```python
from build123d import *

# Parameters (mm, degrees)
F3_DEPTH    = 6.5
F4_T1_DEPTH = 87.9231463955
F4_T3_DEPTH = 86.4923799402
F5_R        = 35
F6_T        = -1.25


# Not quite as in the source:
# - a fillet or chamfer that OpenCascade refuses, or shapes differently, is made with other operations: its cross-section is extruded or revolved along the edge and cut away or added


with BuildPart() as f3:
    # F2 (on Front) → F3 (new body)
    with BuildSketch(Plane.XZ):
        Polygon((0, 19.5199243858), (20, 0), (215, 0), (215, 7.5), (23.0533679898, 7.5), (0, 30), align=None)
    extrude(amount=F3_DEPTH)

    # F4: fillet of radius 40 on 2 edges, made by hand

    # F4_s2 → F4_t1 (cut)
    with BuildSketch(Plane.XZ.offset(-40.7115731978)):
        with BuildLine():
            ThreePointArc((8.3460077876, 11.374252339), (21.2020218527, 2.9525310821), (36.2846292791, 0))
            Line((36.2846292791, 0), (20, 0))
            Line((20, 0), (8.3460077876, 11.374252339))
        make_face()
    extrude(amount=F4_T1_DEPTH, mode=Mode.SUBTRACT)

    # F4_s4 → F4_t3 (cut)
    with BuildSketch(Plane.XZ.offset(-39.9961899701)):
        with BuildLine():
            ThreePointArc((11.4492084149, 8.345540259), (4.0262452257, 18.2748088699), (0, 30))
            Line((0, 30), (0, 19.5199243858))
            Line((0, 19.5199243858), (11.4492084149, 8.345540259))
        make_face()
    extrude(amount=F4_T3_DEPTH, mode=Mode.SUBTRACT)

    # F5
    f5_edges = [f3.edges().sort_by_distance(p)[0] for p in [
        (23.053368, -3.25, 7.5),
    ]]
    fillet(f5_edges, radius=F5_R)

    # F6
    f6_openings = [f3.faces().sort_by_distance(p)[0] for p in [
        (6.428062, -3.25, 23.726235),
        (24.105137, -3.25, 10.083465),
        (126.151209, -3.25, 7.5),
        (215, -3.25, 3.75),
    ]]
    offset(amount=F6_T, openings=f6_openings)


solid = f3.part
```
Build history of the part. All positions in model axes, mm. A direction names the side the tool comes from. Round coordinates to 2 decimals unless told otherwise and drop trailing zeros. Write each loop counter-clockwise with the first axis right and the second up, starting at its lowest first coordinate (ties: lowest second). Pieces come first, ordered by that corner, then holes. Notation, with made-up numbers: (89, -17.5) - (147, -17.5) arc R16 ccw to (147, -12.5) - close; hole circle Ø8 at (-26.5, 65.25). An arc over 180 degrees is marked (long way). Write each question's results on one line, items separated by ' | '. Start each with the question number.
Item 1: Saw through at A-A (x = 93). Write the cut outline in (y, z), and give its area (4 significant figures).
Item 2: Wall check: L1, parallel to Z at x = 160, y = -2; L2, parallel to Z at x = 69, y = -0.5; L3, parallel to X at y = -5.5, z = 13. Give the ranges that are in metal, low to high. Write a range as [from, to].
Item 3: Drop flat-ended pins along their axis: P1, Ø0.6, axis at x = 130, y = -6, coming from the +Z side; P2, Ø1.2, axis at x = 105, y = -3.5, coming from the +Z side; P3, Ø3, axis at y = -4, z = 22.5, coming from the -X side. Give the stop position or say it passes through.
Item 4: Saw through at B-B (y = -4.25). Write the cut outline in (x, z).
Item 5: Mould opens along Y. For faces 1 (the face through (215, -3, 1)), 2 (the face through (108, -1.25, 5)), 3 (the face through (107, 0, 5)) say: pulls with the +Y half, pulls with the -Y half, needs draft (parallel to the pull), parting line crosses it, or undercut.
Item 6: Which spindle directions (+Z, -Z, +X, -X, +Y, -Y) get a long thin tool onto all of the face, cutting with end or side? Do faces 4 (the face through (124, -3, 0)), 5 (the face through (22.502, -3.222, 3.784)). Say none if no direction does.
Results are:
1) outline: (-6.5, 0) - (0, 0) - (0, 7.5) - (-1.25, 7.5) - (-1.25, 1.25) - (-5.25, 1.25) - (-5.25, 7.5) - (-6.5, 7.5) - close | area: 23.75 mm²
2) L1: z = [0, 1.25] | L2: z = [0, 7.5] | L3: x = [7.37, 18.47]
3) P1: stops at z = 7.5 | P2: stops at z = 1.25 | P3: stops at x = 1.55
4) outline: (0, 30) arc R40 ccw to (9.94, 9.9) arc R40 ccw to (36.28, 0) - (215, 0) - (215, 1.25) - (36.28, 1.25) arc R38.75 cw to (10.81, 10.8) arc R38.75 cw to (1.59, 28.45) - close
5) face 1: needs draft | face 2: undercut | face 3: pulls with the +Y half
6) face 4: -Z, +X, -X, +Y, -Y | face 5: +Z, +X
